The model under review builds one solid part; all positions refer to its coordinate system, in mm. Face numbers are marked on the shaded views. A direction names the side the tool comes from. Round coordinates to 2 decimals unless told otherwise and drop trailing zeros. Order: outer loops, then holes, each group sorted by start corner. A loop starts at its lowest first (then second) coordinate and runs counter-clockwise, first axis right, second up. Notation, with made-up numbers: M 60.5,-17.75 L 106.5,-17.75 A8 cw 106.5,-10.75 Z; hole C 83.5,7.5 d4. An arc over 180 degrees is marked long. Answer as a JSON object with one key per item and string values. Group by question number.
1) Insertion check: pin 1 Ø4 at (x, z) = (13.95, 13.95) entering from +Y; pin 2 Ø10 at (y, z) = (28.5, 57.5) entering from +X; pin 3 Ø1.5 at (x, y) = (3.5, 33.5) entering from -Z. Each pin has a flat end and moves straight along its axis. Give the tip position at first contact, or say it passes through.
2) Consider section A-A, the plane x = 0. Write out the cut boundary in (y, z).
3) The part is to be moulded in two halves that separate along Z. For the marked faces 3, 4 and 5, say which applies: +Z half, -Z half, draft (parallel to the pull), parting line (faces both ways), or undercut.
4) For the marked faces 1 and 2, list the 3-axis set-ups (+Z, -Z, +X, -X, +Y, -Y) from which the entire face can be reached by the end or side of a thin tool; tool diameter is ignored.
5) To check wall thickness, follow line 1 (X direction, y = -2.15, z = -13.95) (3 decimals); line 2 (Z direction, x = -7, y = 30.5); line 3 (X direction, y = -2, z = -13). State the ranges of each line that lie inside material, in increasing order.
6) Consider section C-C, the plane z = -43. Write out the cut boundary in (x, y), then the cut area to 3 significant figures.
7) Consider section D-D, the plane x = 35.5. Write out the cut boundary in (y, z), then the cut area to 3 significant figures.
8) Consider section B-B, the plane y = 24. Write out the cut boundary in (x, z).
```python
from build123d import *

# Parameters (mm, degrees)
SKETCH1_R               = 9
SKETCH1_R_2             = 1.225
BOSS_EXTRUDE1_DEPTH     = 3
BOSS_EXTRUDE2_DEPTH     = 38.5
BOSS_EXTRUDE4_DEPTH     = 50
SKETCH2_R               = 2
CUT_EXTRUDE1_DEPTH      = 5
MIRROR2_COPY_1_SKETCH_R = 2
MIRROR2_COPY_1_DEPTH    = 5
MIRROR2_COPY_2_SKETCH_R = 2
MIRROR2_COPY_2_DEPTH    = 5


with BuildPart() as part:
    # Sketch1 → Boss-Extrude1 (new body)
    with BuildSketch(Plane(origin=(0, 0, 0), x_dir=(1, 0, 0), z_dir=(0, 1, 0))):
        Polygon((75, 0), (-37.5, 64.951905284), (-37.5, -64.951905284), align=None)
        with Locations(Location((0, 0, 0), (0, 0, 270))):
            Circle(SKETCH1_R, mode=Mode.SUBTRACT)
        with Locations(Location((-13.95, 13.95, 0), (0, 0, 270))):
            Circle(SKETCH1_R_2, mode=Mode.SUBTRACT)
        with Locations(Location((13.95, 13.95, 0), (0, 0, 270))):
            Circle(SKETCH1_R_2, mode=Mode.SUBTRACT)
        with Locations(Location((13.95, -13.95, 0), (0, 0, 270))):
            Circle(SKETCH1_R_2, mode=Mode.SUBTRACT)
        with Locations(Location((-13.95, -13.95, 0), (0, 0, 270))):
            Circle(SKETCH1_R_2, mode=Mode.SUBTRACT)
    extrude(amount=-BOSS_EXTRUDE1_DEPTH)

    # Sketch1_3 → Boss-Extrude2 (add)
    # profile 1 of 10: a face of its own
    with BuildSketch(Plane(origin=(0, 0, 0), x_dir=(1, 0, 0), z_dir=(0, 1, 0))):
        Polygon((-37.5, 64.951905284), (-37.5, -64.951905284), (75, 0), align=None)
        Polygon((-34.5, -59.755752861), (69, 0), (-34.5, 59.755752861), align=None, mode=Mode.SUBTRACT)
    # profile 2 of 10: a face of its own
    with BuildSketch(Plane(origin=(0, 0, 0), x_dir=(1, 0, 0), z_dir=(0, 1, 0))):
        Polygon((-30.5, 52.827549631), (-34.5, 50.518148554), (-34.5, 47.054046939), (-30.5, 49.363448016), align=None)
    # profile 3 of 10: a face of its own
    with BuildSketch(Plane(origin=(0, 0, 0), x_dir=(1, 0, 0), z_dir=(0, 1, 0))):
        Polygon((-27.5, 51.095498823), (-30.5, 52.827549631), (-30.5, 49.363448016), align=None)
    # profile 4 of 10: a face of its own
    with BuildSketch(Plane(origin=(0, 0, 0), x_dir=(1, 0, 0), z_dir=(0, 1, 0))):
        Polygon((-26.5, 55.136950708), (-30.5, 52.827549631), (-27.5, 51.095498823), (-23.5, 53.4048999), align=None)
    # profile 5 of 10: a face of its own
    with BuildSketch(Plane(origin=(0, 0, 0), x_dir=(1, 0, 0), z_dir=(0, 1, 0))):
        Polygon((58, 6.350852961), (58, 1.732050808), (61, 0), (61, 4.618802154), align=None)
    # profile 6 of 10: a face of its own
    with BuildSketch(Plane(origin=(0, 0, 0), x_dir=(1, 0, 0), z_dir=(0, 1, 0))):
        Polygon((61, 0), (58, 1.732050808), (58, -1.732050808), align=None)
    # profile 7 of 10: a face of its own
    with BuildSketch(Plane(origin=(0, 0, 0), x_dir=(1, 0, 0), z_dir=(0, 1, 0))):
        Polygon((61, -4.618802154), (61, 0), (58, -1.732050808), (58, -6.350852961), align=None)
    # profile 8 of 10: a face of its own
    with BuildSketch(Plane(origin=(0, 0, 0), x_dir=(1, 0, 0), z_dir=(0, 1, 0))):
        Polygon((-30.5, -49.363448016), (-34.5, -47.054046939), (-34.5, -50.518148554), (-30.5, -52.827549631), align=None)
    # profile 9 of 10: a face of its own
    with BuildSketch(Plane(origin=(0, 0, 0), x_dir=(1, 0, 0), z_dir=(0, 1, 0))):
        Polygon((-27.5, -51.095498823), (-30.5, -52.827549631), (-26.5, -55.136950708), (-23.5, -53.4048999), align=None)
    # profile 10 of 10: a face of its own
    with BuildSketch(Plane(origin=(0, 0, 0), x_dir=(1, 0, 0), z_dir=(0, 1, 0))):
        Polygon((-27.5, -51.095498823), (-30.5, -49.363448016), (-30.5, -52.827549631), align=None)
    extrude(amount=BOSS_EXTRUDE2_DEPTH)

    # Sketch1_5 → Boss-Extrude4 (add)
    with BuildSketch(Plane(origin=(0, 0, 0), x_dir=(1, 0, 0), z_dir=(0, 1, 0))):
        Polygon((58, 1.732050808), (-27.5, 51.095498823), (-30.5, 49.363448016), (-30.5, -49.363448016), (-27.5, -51.095498823), (58, -1.732050808), align=None)
        Polygon((-27.5, 47.631397208), (55, 0), (-27.5, -47.631397208), align=None, mode=Mode.SUBTRACT)
    extrude(amount=BOSS_EXTRUDE4_DEPTH)

    # Sketch2 → Cut-Extrude1 (cut, symmetric)
    with BuildSketch(Plane(origin=(-5.024047358, 0, 8.701905284), x_dir=(0.4999999999999999, 0, -0.8660254037844386), z_dir=(0.8660254037844387, 0, 0.49999999999999994))):
        with Locations((-59.951905284, 33.5)):
            Circle(SKETCH2_R)
    cut_extrude1 = extrude(amount=CUT_EXTRUDE1_DEPTH, both=True, mode=Mode.SUBTRACT)

    # Mirror1: Cut-Extrude1 across plane
    add(cut_extrude1.mirror(Plane(origin=(0, 0, 0), x_dir=(0.5000000000000001, 0, 0.8660254037844387), z_dir=(-0.8660254037844388, 0, 0.49999999999999994))), mode=Mode.SUBTRACT)

    # Mirror2 copy 1 sketch → Mirror2 copy 1 (cut, symmetric)
    with BuildSketch(Plane(origin=(10.048094716, 0, 0), x_dir=(-1, 0, 0), z_dir=(0, 0, -1))):
        with Locations((-59.951905284, 33.5)):
            Circle(MIRROR2_COPY_1_SKETCH_R)
    extrude(amount=MIRROR2_COPY_1_DEPTH, both=True, mode=Mode.SUBTRACT)

    # Mirror2 copy 2 sketch → Mirror2 copy 2 (cut, symmetric)
    with BuildSketch(Plane(origin=(-5.024047358, 0, -8.701905284), x_dir=(0.4999999999999999, 0, 0.8660254037844386), z_dir=(0.8660254037844387, 0, -0.49999999999999994))):
        with Locations((-59.951905284, -33.5)):
            Circle(MIRROR2_COPY_2_SKETCH_R)
    extrude(amount=MIRROR2_COPY_2_DEPTH, both=True, mode=Mode.SUBTRACT)


solid = part.part
```
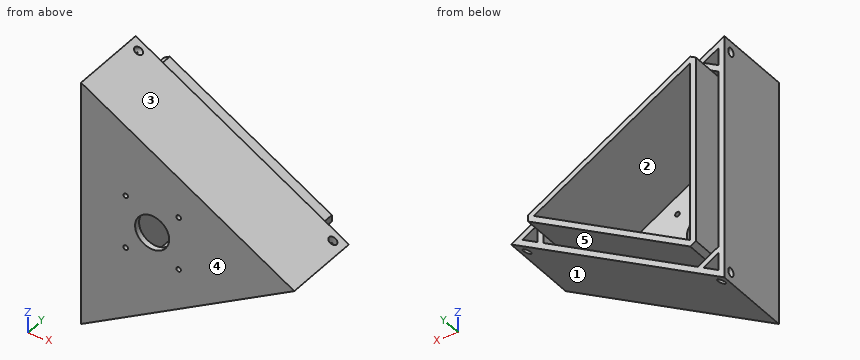
Results list:
{
 "1": {"pin 1": "y = 0", "pin 2": "x = -15.93", "pin 3": "z = -41.71"},
 "2": {"outline": "M -3,-43.3 L 38.5,-43.3 L 38.5,-39.84 L 0,-39.84 L 0,-35.22 L 50,-35.22 L 50,-31.75 L 0,-31.75 L 0,-9 L -3,-9 Z; M -3,9 L 0,9 L 0,31.75 L 50,31.75 L 50,35.22 L 0,35.22 L 0,39.84 L 38.5,39.84 L 38.5,43.3 L -3,43.3 Z"},
 "3": {"face 3": "+Z half", "face 4": "draft", "face 5": "undercut"},
 "4": {"face 1": "-Z, +X, +Y, -Y", "face 2": "+Y"},
 "5": {"line 1": "-37.5 to -15.175, -12.725 to 12.725, 15.175 to 50.838", "line 2": "-47.34 to -43.88, -39.26 to -35.8, 35.8 to 39.26, 43.88 to 47.34", "line 3": "-37.5 to -14.72, -13.18 to 13.18, 14.72 to 52.48"},
 "6": {"outline": "M -37.5,-3 L 0.52,-3 L 0.52,38.5 L -5.48,38.5 L -5.48,0 L -13.48,0 L -13.48,50 L -19.48,50 L -19.48,0 L -27.5,0 L -27.5,50 L -30.5,50 L -30.5,0 L -34.5,0 L -34.5,38.5 L -37.5,38.5 Z", "area": "911 mm^2"},
 "7": {"outline": "M -3,-22.81 L 38.5,-22.81 L 38.5,-19.34 L 0,-19.34 L 0,-14.72 L 50,-14.72 L 50,-11.26 L 0,-11.26 L 0,11.26 L 50,11.26 L 50,14.72 L 0,14.72 L 0,19.34 L 38.5,19.34 L 38.5,22.81 L -3,22.81 Z", "area": "750 mm^2"},
 "8": {"outline": "M -37.5,-64.95 L 75,0 L -37.5,64.95 Z; hole M -34.5,-59.76 L -26.5,-55.14 L -34.5,-50.52 Z; hole M -34.5,-47.05 L -30.5,-49.36 L -30.5,49.36 L -34.5,47.05 Z; hole M -34.5,50.52 L -26.5,55.14 L -34.5,59.76 Z; hole M -27.5,-51.1 L -23.5,-53.4 L 58,-6.35 L 58,-1.73 Z; hole M -27.5,-47.63 L 55,0 L -27.5,47.63 Z; hole M -27.5,51.1 L 58,1.73 L 58,6.35 L -23.5,53.4 Z; hole M 61,-4.62 L 69,0 L 61,4.62 Z"}
}
